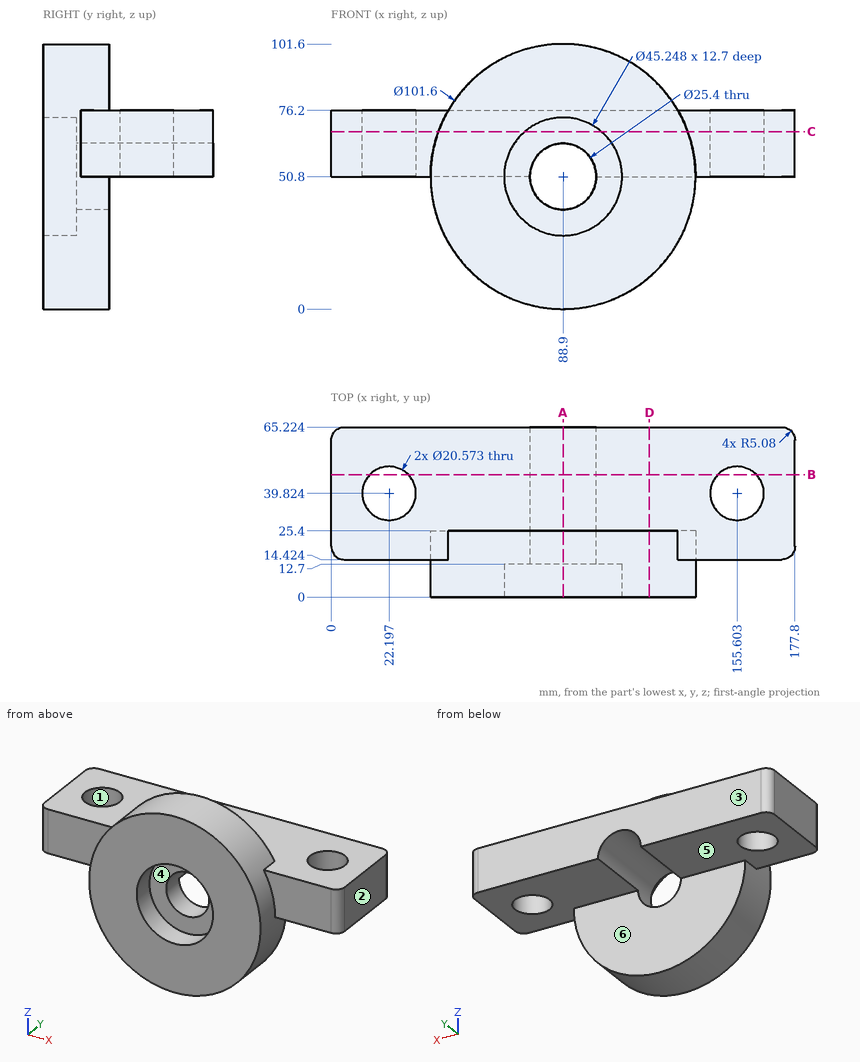
Input: dimensioned drawing with shaded views. Units: mm. Origin: part minimum x, y, z. A direction names the side the tool comes from. Coordinates: 2 decimals unless noted, no trailing zeros. Write each loop counter-clockwise with the first axis right and the second up, starting at its lowest first coordinate (ties: lowest second). Pieces come first, ordered by that corner, then holes. Notation, with made-up numbers: M -14.75,-21.5 L 9.25,-21.5 A9 cw 9.25,-5.5 Z; hole C -21,57 d3. An arc over 180 degrees is marked long. Answer as CSV lines item,"result". Start each with the question number.
Q1. Mould query, pull axis X, two halves, no side actions, for the marked faces 1, 2 and 3. Classes: released by +X, released by -X, zero draft, split by the parting line, or undercut.
Q2. Reachability of the marked faces 4, 5 and 6 from +Z, -Z, +X, -X, +Y, -Y: full face, straight path, thin tool, end or side. Return the list, or none.
Q3. Cut plane D-D on x = 122. Return the cut outline in (y, z).
Q4. Cut plane A-A on x = 88.9. Return the cut outline in (y, z), then the cut area to 3 significant figures.
Q5. Cut plane C-C on z = 68. Return the cut outline in (x, y).
Q6. Cut plane B-B on y = 47. Return the cut outline in (x, z), then the cut area to 3 significant figures.
Q7. Line query: line 1 (Z direction, x = 88, y = 10) (1 decimal); line 2 (Z direction, x = 145, y = 44.5); line 3 (X direction, y = 9, z = 50). Output: solid intervals per line, ascending. Write a range as from..to.
Q8. Pin query (flat end, axial travel): P1, Ø15, axis at x = 120.5, y = 49.5, coming from the +Z side; P2, Ø6, axis at x = 87.5, y = 20, coming from the -Z side; P3, Ø10, axis at x = 37.5, y = 49.5, coming from the -Z side. Return the tip coordinate at first contact, or that it passes through.
Findings below:
1,face 1,"undercut"
1,face 2,"released by +X"
1,face 3,"zero draft"
2,face 4,"-Y"
2,face 5,"-Z, -X, +Y"
2,face 6,"-Z, +X, -X, +Y"
3,outline,"M 0,12.26 L 25.4,12.26 L 25.4,50.8 L 65.22,50.8 L 65.22,76.2 L 25.4,76.2 L 25.4,89.34 L 0,89.34 Z"
4,outline,"M 0,0 L 25.4,0 L 25.4,38.1 L 12.7,38.1 L 12.7,28.18 L 0,28.18 Z; M 0,73.42 L 12.7,73.42 L 12.7,63.5 L 65.22,63.5 L 65.22,76.2 L 25.4,76.2 L 25.4,101.6 L 0,101.6 Z"
4,area,"2,190 mm2"
5,outline,"M 0,19.5 A5.08 ccw 5.08,14.42 L 41.1,14.42 L 41.1,0 L 74.2,0 L 74.2,12.7 L 103.6,12.7 L 103.6,0 L 136.7,0 L 136.7,14.42 L 172.72,14.42 A5.08 ccw 177.8,19.5 L 177.8,60.14 A5.08 ccw 172.72,65.22 L 5.08,65.22 A5.08 ccw 0,60.14 Z; hole C 22.2,39.82 d20.57; hole C 155.6,39.82 d20.57"
6,outline,"M 0,50.8 L 14.83,50.8 L 14.83,76.2 L 0,76.2 Z; M 29.57,50.8 L 76.2,50.8 A12.7 cw 101.6,50.8 L 148.23,50.8 L 148.23,76.2 L 29.57,76.2 Z; M 162.97,50.8 L 177.8,50.8 L 177.8,76.2 L 162.97,76.2 Z"
6,area,"3,510 mm2"
7,line 1,"z = 0..28.2, 73.4..101.6"
7,line 2,"z = 50.8..76.2"
7,line 3,"x = 38.11..66.29, 111.51..139.69"
8,P1,"stops at z = 76.2"
8,P2,"stops at z = 0"
8,P3,"stops at z = 50.8"
